Design review of the part built by this model. Coordinates are the model's own, in mm. A direction names the side the tool comes from. Round coordinates to 2 decimals unless told otherwise and drop trailing zeros. Loops run counter-clockwise (first coordinate to the right, second up) from the corner with the lowest first, then second, coordinate; pieces in that order, holes last. Notation, with made-up numbers: (49.5, -21) -> (55.5, -21) arc R10 ccw to (55.5, -14) -> close; hole circle Ø9 at (30.5, 9.5). An arc over 180 degrees is marked (long way). Answer as CSV lines item,"result". Start each with the question number.
Autodesk Inventor part; units mm, degrees
ref_plane "YZ Plane" through (0, 0, 0) normal (1, 0, 0) x (0, 1, 0)
ref_plane "XZ Plane" through (0, 0, 0) normal (0, 1, 0) x (-1, 0, 0)
ref_plane "XY Plane" through (0, 0, 0) normal (0, 0, 1) x (1, 0, 0)
sketch "Sketch1" plane through (0, 0, 0) normal (1, 0, 0) x (0, 1, 0)
  line L0 (-28.75, 25) -> (28.75, 25)
  line L1 (28.75, 25) -> (28.75, -25)
  line L2 (28.75, -25) -> (-28.75, -25)
  line L3 (-28.75, -25) -> (-28.75, 25)
  line L4 (-28.75, 25) -> (28.75, -25) construction
  line L5 (28.75, 25) -> (-28.75, -25) construction
  point P0 (0, 0)
  dimension "d0" = 57.5
  dimension "d1" = 50
extrude "Extrusion1" add sketch "Sketch1" along normal blind 3
sketch "Sketch4" plane through (0, -28.75, 25) normal (0, 0, 1) x (1, 0, 0)
  line L0 (0, 0) -> (0, 57.5)
  arc A0 (0, 54.5) -> (0, 44.5) centre (0, 49.5) ccw
  line L1 (-0.8, 44.5644) -> (-0.8, 46.0644)
  line L2 (-0.8, 46.0644) -> (-2.3, 46.0644)
  line L3 (-2.3, 46.0644) -> (-2.3, 45.0604)
  line L4 (-5, 49.5) -> (0, 49.5) construction
  line L5 (-0.8, 54.4356) -> (-0.8, 52.9356)
  line L6 (-0.8, 52.9356) -> (-2.3, 52.9356)
  line L7 (-2.3, 52.9356) -> (-2.3, 53.9396)
  line L8 (0, 0) -> (3, 0)
  arc A1 (0, 13) -> (0, 3) centre (0, 8) ccw
  line L9 (-0.8, 3.0644) -> (-0.8, 4.5644)
  line L10 (-0.8, 4.5644) -> (-2.3, 4.5644)
  line L11 (-2.3, 4.5644) -> (-2.3, 3.5604)
  line L12 (-5, 8) -> (0, 8) construction
  line L13 (-0.8, 12.9356) -> (-0.8, 11.4356)
  line L14 (-0.8, 11.4356) -> (-2.3, 11.4356)
  line L15 (-2.3, 11.4356) -> (-2.3, 12.4396)
  point P0 (0, 28.75)
  point P1 (-2.3, 53.9396)
  dimension "d15" = 1.5
  dimension "d16" = 1.5
  dimension "d17" = 0.8
  dimension "d25" = 3
  dimension "d26" = 10
  dimension "d28" = 1.5
  dimension "d31" = 10
  dimension "d32" = 3
  dimension "d33" = 1.5
extrude "Extrusion3" add sketch "Sketch4" against normal blind 49 contours A0 L1 L2 L3 L7 L6 L5 L0
fillet "Fillet2" radius 2 1 edges at (3, 28.75, 0)
extrude "Extrusion4" add sketch "Sketch4" against normal blind 49 contours A1 L9 L10 L11 L15 L14 L13 L0
properties part number "Cover of Sensors_3DPrint"
Q1. Add section B-B, the plane z = -2. Give the boundary of the cut face in (x, y).
Q2. Add section C-C, the plane y = 1. Give the boundary of the cut face in (x, z).
Q3. Machinability: for faces 5 (the flat face through (-0.8, -17, 1)), 6 (the flat face through (-0.8, 25, 1)), 7 (the flat face through (-2, -21, -24)), which of the approach directions +Z, -Z, +X, -X, +Y, -Y give a long, thin tool a straight path to every point of the face, cutting with its end or side? Answer none if there is none.
Q4. To check wall thickness, follow probe 1 along Y at (x, z) = (-0.75, -4); probe 2 along Y at (x, z) = (-2, 15.5); probe 3 along X at (y, z) = (-6, -13.5). State the ranges of each line that lie inside material, in increasing order. Write a range as from..to.
Q5. For pin 1 Ø0.8 at (y, z) = (-16.5, -6.5) entering from -X; pin 2 Ø15 at (y, z) = (-8, 0) entering from -X; pin 3 Ø3 at (x, y) = (-3, 5.5) entering from -Z; pin 4 Ø1.2 at (y, z) = (16.5, -4.5) entering from -X, all flat-tipped, find the tip position at first contact; note any pin that passes through.
Q6. Mouldability with a two-part tool opening along Y and no side actions: class faces 1 (the cylindrical face through (2.4, 28.18, -0.35)), 2 (the flat face through (1, -28.75, 0)), 3 (the flat face through (-2, 21, -24)), 4 (the cylindrical face through (-5, 20.8, 0.8)) as pulls with the +Y half, pulls with the -Y half, needs draft (parallel to the pull), parting line crosses it, or undercut.
Q7. Add section D-D, the plane y = -22. Give the boundary of the cut face in (x, z), and give its area (3 significant figures).
Q8. Add section A-A, the plane x = -4. Give the boundary of the cut face in (y, z).
Worked answers:
1,outline,"(-2.3, -25.19) -> (-2.3, -24.19) -> (-0.8, -24.19) -> (-0.8, -25.69) arc R5 ccw to (0, -25.75) -> (0, -28.75) -> (3, -28.75) -> (3, 26.75) arc R2 ccw to (1, 28.75) -> (0, 28.75) -> (0, 25.75) arc R5 ccw to (-0.8, 25.69) -> (-0.8, 24.19) -> (-2.3, 24.19) -> (-2.3, 25.19) arc R5 ccw to (-2.3, 16.31) -> (-2.3, 17.31) -> (-0.8, 17.31) -> (-0.8, 15.81) arc R5 ccw to (0, 15.75) -> (0, -15.75) arc R5 ccw to (-0.8, -15.81) -> (-0.8, -17.31) -> (-2.3, -17.31) -> (-2.3, -16.31) arc R5 ccw to start"
2,outline,"(0, -25) -> (3, -25) -> (3, 25) -> (0, 25) -> close"
3,face 5,"+Z, -Z"
3,face 6,"+Z, -Z, +Y"
3,face 7,"-Z, -X, +Y, -Y"
4,probe 1,"y = -25.69..-15.81, 15.81..25.69"
4,probe 2,"y = -24.19..-17.31, 17.31..24.19"
4,probe 3,"x = 0..3"
5,pin 1,"stops at x = -3.19"
5,pin 2,"stops at x = 0"
5,pin 3,"passes through"
5,pin 4,"stops at x = -3.42"
6,face 1,"pulls with the +Y half"
6,face 2,"pulls with the -Y half"
6,face 3,"needs draft"
6,face 4,"undercut"
7,outline,"(-4.84, -24) -> (0, -24) -> (0, -25) -> (3, -25) -> (3, 25) -> (-4.84, 25) -> close"
7,area,"387 mm^2"
8,outline,"(-23.75, -24) -> (-17.75, -24) -> (-17.75, 25) -> (-23.75, 25) -> close; (17.75, -24) -> (23.75, -24) -> (23.75, 25) -> (17.75, 25) -> close"
